Geometry: final body of the model. Coordinates: model frame, mm. Round coordinates to 2 decimals unless told otherwise and drop trailing zeros. Loops run counter-clockwise (first coordinate to the right, second up) from the corner with the lowest first, then second, coordinate; pieces in that order, holes last. Notation, with made-up numbers: M -1.75,86 L 53.25,86 A8 cw 53.25,97 Z; hole C 57.25,35 d9. An arc over 180 degrees is marked long. Return JSON: item names as keys, results as strings.
from build123d import *

# Parameters (mm, degrees)
BOSS_EXTRUDE3_DEPTH              = 14.5
SKETCH8_R                        = 7.935
CUT_EXTRUDE3_DEPTH               = 88
CUT_EXTRUDE9_DEPTH               = 2.4
F_39_0_13779528_DIAMETER_HOLE1_D = 3.500000112
CUT_EXTRUDE10_DEPTH              = 22.4
CUT_EXTRUDE11_DEPTH              = 2.4


with BuildPart() as part:
    # Sketch6 → Boss-Extrude3 (new body)
    with BuildSketch(Plane(origin=(0, 0, 0), x_dir=(1, 0, 0), z_dir=(0, 1, 0))):
        Polygon((-16.836914056, 5.783353512), (13.163085944, 5.783353512), (20.663085944, -47.581919406), (-24.336914056, -47.581919406), align=None)
    extrude(amount=BOSS_EXTRUDE3_DEPTH)

    # Sketch8 → Cut-Extrude3 (cut)
    with BuildSketch(Plane.XY.offset(47.581919406)):
        with Locations((-1.836914056, 0)):
            Circle(SKETCH8_R)
    extrude(amount=-CUT_EXTRUDE3_DEPTH, mode=Mode.SUBTRACT)

    # Sketch18 → Cut-Extrude9 (cut)
    with BuildSketch(Plane(origin=(0, 14.5, 0), x_dir=(1, 0, 0), z_dir=(0, 1, 0))):
        Polygon((-15.771819769, -44.868285994), (-12.821819769, -43.1651027), (-12.821819769, -39.758736112), (-15.771819769, -38.055552818), (-18.721819769, -39.758736112), (-18.721819769, -43.1651027), align=None)
        Polygon((12.097991657, -44.868285994), (15.047991657, -43.1651027), (15.047991657, -39.758736112), (12.097991657, -38.055552818), (9.147991657, -39.758736112), (9.147991657, -43.1651027), align=None)
        Polygon((11.389331688, -26.016021021), (14.389331688, -24.283970214), (14.389331688, -20.819868599), (11.389331688, -19.087817791), (8.389331688, -20.819868599), (8.389331688, -24.283970214), align=None)
        Polygon((-15.0631598, -26.016021021), (-12.0631598, -24.283970214), (-12.0631598, -20.819868599), (-15.0631598, -19.087817791), (-18.0631598, -20.819868599), (-18.0631598, -24.283970214), align=None)
    extrude(amount=-CUT_EXTRUDE9_DEPTH, mode=Mode.SUBTRACT)

    # #39 (0.13779528) Diameter Hole1 (through all)
    with Locations(Plane(origin=(-15.0631598, 14.5, 22.551919406), x_dir=(0, 0, 1), z_dir=(0, 1, 0))):
        with Locations((0, 0), (0, 26.452491488), (18.91, -0.708659969), (18.91, 27.161151457)):
            Hole(F_39_0_13779528_DIAMETER_HOLE1_D / 2)

    # Sketch22 → Cut-Extrude10 (cut)
    with BuildSketch(Plane(origin=(0, 14.5, 0), x_dir=(1, 0, 0), z_dir=(0, 1, 0))):
        Polygon((-22.781301734, -36.51316259), (19.107473622, -36.51316259), (13.163085944, 5.783353512), (-16.836914056, 5.783353512), align=None)
    extrude(amount=-CUT_EXTRUDE10_DEPTH, mode=Mode.SUBTRACT)

    # Sketch24 → Cut-Extrude11 (cut)
    with BuildSketch(Plane.XZ):
        Polygon((-15.771819769, 38.055552818), (-12.821819769, 39.758736112), (-12.821819769, 43.1651027), (-15.771819769, 44.868285994), (-18.721819769, 43.1651027), (-18.721819769, 39.758736112), align=None)
        Polygon((12.097991657, 38.055552818), (15.047991657, 39.758736112), (15.047991657, 43.1651027), (12.097991657, 44.868285994), (9.147991657, 43.1651027), (9.147991657, 39.758736112), align=None)
    extrude(amount=-CUT_EXTRUDE11_DEPTH, mode=Mode.SUBTRACT)


solid = part.part
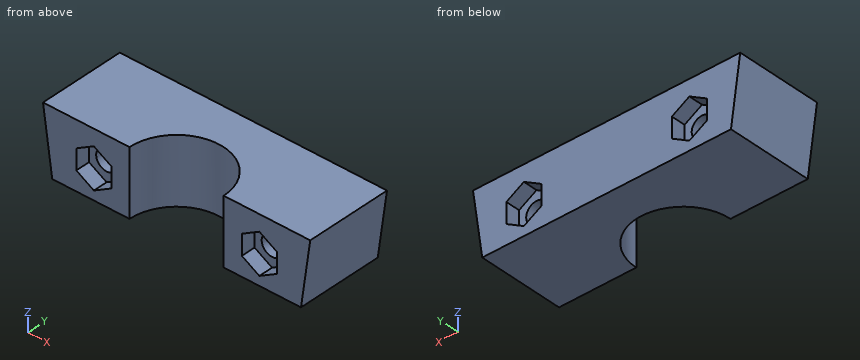
Q1. Pin query (flat end, axial travel): pin 1 (6 mm diameter, centred on x = -1, z = 40.5, fed in from -Y); pin 2 (6 mm diameter, centred on y = 12, z = 45.5, fed in from -X); pin 3 (1.9 mm diameter, centred on y = 1.5, z = 41, fed in from -X). Return the tip coordinate at first contact, or that it passes through.
Determined:
{"pin 1": "stops at y = 6.95", "pin 2": "stops at x = -24.34", "pin 3": "stops at x = -23.55"}
Q2. Material intervals for L1, parallel to X at y = 9.75, z = 40.75; L2, parallel to X at y = 1.5, z = 39; L3, parallel to X at y = 10.75, z = 40.25, sorted ascending.
Determined:
{"L1": "x = -23.38 to -17.37, -14.17 to 10.5, 13.7 to 19.7", "L2": "x = -23.13 to -17.41, -14.14 to -9.63, 5.96 to 10.46, 13.73 to 19.46", "L3": "x = -23.31 to -17.03, -14.51 to 10.84, 13.36 to 19.63"}
Q3. Section query B-B (y = 3.75). Output: boundary loops of the cut face in (x, z).
Determined:
{"outline": "M -24.34,47.58 L -22.78,36.51 L -8.83,36.51 L -8.83,47.58 Z; M 5.16,36.51 L 19.11,36.51 L 20.66,47.58 L 5.16,47.58 Z; hole C -15.77,41.46 d3.5; hole C 12.1,41.46 d3.5"}
Q4. Section query A-A (y = 12.75). Output: boundary loops of the cut face in (x, z).
Determined:
{"outline": "M -24.34,47.58 L -22.78,36.51 L 19.11,36.51 L 20.66,47.58 Z; hole M -18.72,39.76 L -15.77,38.06 L -12.82,39.76 L -12.82,43.17 L -15.77,44.87 L -18.72,43.17 Z; hole M 9.15,39.76 L 12.1,38.06 L 15.05,39.76 L 15.05,43.17 L 12.1,44.87 L 9.15,43.17 Z"}
Q5. Section query C-C (z = 41). State how many separate pieces and enclosed holes the cut face has, plus the area to 3 significant figures.
Determined:
{"separate pieces": "3", "enclosed holes": "0", "area": "405 mm^2"}
Q6. Section query D-D (x = -17). Output: boundary loops of the cut face in (y, z), plus the area to 3 significant figures.
Determined:
{"outline": "M 0,36.51 L 14.5,36.51 L 14.5,38.76 L 12.1,38.76 L 12.1,40.22 L 2.4,40.22 L 2.4,38.76 L 0,38.76 Z; M 0,44.16 L 2.4,44.16 L 2.4,42.71 L 12.1,42.71 L 12.1,44.16 L 14.5,44.16 L 14.5,47.58 L 0,47.58 Z", "area": "110 mm^2"}
